from build123d import *

# Parameters (mm, degrees)
BOSS_EXTRUDE1_DEPTH               = 38.1
FILLET1_R                         = 5.08
SKETCH8_R                         = 1.7499965
SKETCH8_R_2                       = 1.75
CUT_EXTRUDE2_DEPTH                = 7.62
F_1_8_0_15_DOWEL_HOLE1_AT_2_COUNT = 2
F_1_8_0_15_DOWEL_HOLE1_AT_2_PITCH = 28.575
F_1_8_0_15_DOWEL_HOLE1_AT_3_COUNT = 2
F_1_8_0_15_DOWEL_HOLE1_AT_3_PITCH = 34.925
F_1_8_0_15_DOWEL_HOLE1_AT_4_COUNT = 2
F_1_8_0_15_DOWEL_HOLE1_AT_4_PITCH = 63.5
CUT_EXTRUDE3_DEPTH                = 4.7752
LPATTERN1_COUNT                   = 2
LPATTERN1_PITCH                   = 63.5
LPATTERN1_COUNT_DIR2              = 2
LPATTERN1_PITCH_DIR2              = 25.4
SKETCH16_W                        = 2.54
SKETCH16_H                        = 44.45
CUT_EXTRUDE4_DEPTH                = 7.62
SKETCH17_W                        = 76.2
SKETCH17_H                        = 19.05
CUT_EXTRUDE5_DEPTH                = 4.7752
SKETCH19_W                        = 12.6492
SKETCH19_H                        = 19.05
SKETCH19_W_2                      = 5.0292
BOSS_EXTRUDE6_DEPTH               = 4.7752
SKETCH22_R                        = 3.175
CGTEST1_DEPTH                     = 7.62


with BuildPart() as part:
    # Sketch1 → Boss-Extrude1 (new, symmetric)
    with BuildSketch(Plane.XY):
        Polygon((0, -24.348466848), (0, 114.923832009), (10.16, 114.923832009), (10.16, 122.543832009), (10.16, 142.863832009), (2.54, 142.863832009), (2.54, 122.543832009), (-7.62, 122.543832009), (-7.62, 114.923832009), (-7.62, -31.968466848), (2.54, -31.968466848), (2.54, -52.288466848), (10.16, -52.288466848), (10.16, -31.968466848), (10.16, -24.348466848), align=None)
    extrude(amount=BOSS_EXTRUDE1_DEPTH, both=True)

    # Fillet1
    fillet1_edges = [part.edges().sort_by_distance(p)[0] for p in [
        (0, -24.348466848, 0),
        (2.54, -31.968466848, 0),
        (0, 114.923832009, 0),
        (2.54, 122.543832009, 0),
        (-7.62, 122.543832009, 0),
        (-7.62, -31.968466848, 0),
    ]]
    fillet(fillet1_edges, radius=FILLET1_R - 0.0001)  # a hair under: the kernel refuses the full size

    # Sketch8 → Cut-Extrude2 (cut)
    with BuildSketch(Plane.ZY.offset(-2.54)):
        with Locations(Location((-31.75, 135.243832009, 0), (0, 0, 270))):
            Circle(SKETCH8_R)
        with Locations(Location((31.75, 135.243832009, 0), (0, 0, 270))):
            Circle(SKETCH8_R)
        with Locations(Location((-10.583333333, 135.243832009, 0), (0, 0, 270))):
            Circle(SKETCH8_R_2)
        with Locations(Location((10.583333333, 135.243832009, 0), (0, 0, 270))):
            Circle(SKETCH8_R_2)
    cut_extrude2 = extrude(amount=-CUT_EXTRUDE2_DEPTH, mode=Mode.SUBTRACT)

    # Mirror1: Cut-Extrude2 across plane
    add(cut_extrude2.mirror(Plane.ZX.offset(45.28768258)), mode=Mode.SUBTRACT)

    # Sketch11 → 1/8 (0.15) Dowel Hole1 (revolve, cut)
    with BuildSketch(Plane(origin=(-7.62, 27.82518258, 12.7), x_dir=(0, 0, 1), z_dir=(0, 1, 0))):
        Polygon((0, 0), (0, 8.764639479), (1.905, 7.62), (1.905, 0), align=None)
    f_1_8_0_15_dowel_hole1 = revolve(axis=Axis((-13.97, 27.82518258, 12.7), (1, 0, 0)), mode=Mode.SUBTRACT)

    # 1/8 (0.15) Dowel Hole1 at 2: 1/8 (0.15) Dowel Hole1 ×2
    with Locations(*[(0, -i * F_1_8_0_15_DOWEL_HOLE1_AT_2_PITCH, 0) for i in range(1, F_1_8_0_15_DOWEL_HOLE1_AT_2_COUNT)]):
        add(f_1_8_0_15_dowel_hole1, mode=Mode.SUBTRACT)

    # 1/8 (0.15) Dowel Hole1 at 3: 1/8 (0.15) Dowel Hole1 ×2
    with Locations(*[(0, i * F_1_8_0_15_DOWEL_HOLE1_AT_3_PITCH, 0) for i in range(1, F_1_8_0_15_DOWEL_HOLE1_AT_3_COUNT)]):
        add(f_1_8_0_15_dowel_hole1, mode=Mode.SUBTRACT)

    # 1/8 (0.15) Dowel Hole1 at 4: 1/8 (0.15) Dowel Hole1 ×2
    with Locations(*[(0, i * F_1_8_0_15_DOWEL_HOLE1_AT_4_PITCH, 0) for i in range(1, F_1_8_0_15_DOWEL_HOLE1_AT_4_COUNT)]):
        add(f_1_8_0_15_dowel_hole1, mode=Mode.SUBTRACT)

    # Sketch14 → Cut-Extrude3 (cut)
    with BuildSketch(Plane.ZY.offset(7.62)):
        Polygon((13.9954, 95.427086941), (11.4046, 95.427086941), (10.1092, 94.136177076), (10.1092, 59.947777076), (11.400109865, 58.652377076), (12.7, 58.652377076), (13.999890135, 58.652377076), (15.2908, 59.947777076), (15.2908, 94.136177076), align=None)
    cut_extrude3 = extrude(amount=-CUT_EXTRUDE3_DEPTH, mode=Mode.SUBTRACT)

    # LPattern1: Cut-Extrude3 2 × 2
    with Locations(*[(0, -i * LPATTERN1_PITCH, -j * LPATTERN1_PITCH_DIR2) for i in range(LPATTERN1_COUNT) for j in range(LPATTERN1_COUNT_DIR2) if (i, j) != (0, 0)]):
        add(cut_extrude3, mode=Mode.SUBTRACT)

    # Mirror2: 1/8 (0.15) Dowel Hole1 across plane
    add(f_1_8_0_15_dowel_hole1.mirror(Plane.XY), mode=Mode.SUBTRACT)

    # Mirror2 copy 1 sketch → Mirror2 copy 1 (revolve, cut)
    with BuildSketch(Plane(origin=(-7.62, -0.74981742, -12.7), x_dir=(0, 0, -1), z_dir=(0, 1, 0))):
        Polygon((0, 0), (0, -8.764639479), (1.905, -7.62), (1.905, 0), align=None)
    revolve(axis=Axis((-13.97, -0.74981742, -12.7), (-1, 0, 0)), mode=Mode.SUBTRACT)

    # Mirror2 copy 2 sketch → Mirror2 copy 2 (revolve, cut)
    with BuildSketch(Plane(origin=(-7.62, 62.75018258, -12.7), x_dir=(0, 0, -1), z_dir=(0, 1, 0))):
        Polygon((0, 0), (0, -8.764639479), (1.905, -7.62), (1.905, 0), align=None)
    revolve(axis=Axis((-13.97, 62.75018258, -12.7), (-1, 0, 0)), mode=Mode.SUBTRACT)

    # Mirror2 copy 3 sketch → Mirror2 copy 3 (revolve, cut)
    with BuildSketch(Plane(origin=(-7.62, 91.32518258, -12.7), x_dir=(0, 0, -1), z_dir=(0, 1, 0))):
        Polygon((0, 0), (0, -8.764639479), (1.905, -7.62), (1.905, 0), align=None)
    revolve(axis=Axis((-13.97, 91.32518258, -12.7), (-1, 0, 0)), mode=Mode.SUBTRACT)

    # Sketch16 → Cut-Extrude4 (cut)
    with BuildSketch(Plane.ZY.offset(7.62)):
        with Locations((3.81, 77.03768258)):
            Rectangle(SKETCH16_W, SKETCH16_H)
    cut_extrude4 = extrude(amount=-CUT_EXTRUDE4_DEPTH, mode=Mode.SUBTRACT)

    # Sketch17 → Cut-Extrude5 (cut)
    with BuildSketch(Plane.ZY.offset(7.62)):
        with Locations((0, 77.03768258)):
            Rectangle(SKETCH17_W, SKETCH17_H)
    cut_extrude5 = extrude(amount=-CUT_EXTRUDE5_DEPTH, mode=Mode.SUBTRACT)

    # Sketch19 → Boss-Extrude6 (add)
    with BuildSketch(Plane.ZY.offset(2.8448)):
        with Locations((-3.7846, 77.03768258)):
            Rectangle(SKETCH19_W, SKETCH19_H)
        with Locations((7.5946, 77.03768258)):
            Rectangle(SKETCH19_W_2, SKETCH19_H)
    boss_extrude6 = extrude(amount=BOSS_EXTRUDE6_DEPTH)

    # Mirror3: Cut-Extrude4, Cut-Extrude5, Boss-Extrude6 across plane
    add(cut_extrude4.mirror(Plane.ZX.offset(45.28768258)), mode=Mode.SUBTRACT)
    add(cut_extrude5.mirror(Plane.ZX.offset(45.28768258)), mode=Mode.SUBTRACT)
    add(boss_extrude6.mirror(Plane.ZX.offset(45.28768258)))

    # Sketch22 → CGTest1 (cut)
    with BuildSketch(Plane.ZY.offset(-2.54)):
        with Locations(Location((0, 135.243832009, 0), (0, 0, 270))):
            Circle(SKETCH22_R)
    extrude(amount=-CGTEST1_DEPTH, mode=Mode.SUBTRACT)


solid = part.part
Geometry: final body of the model. Coordinates: model frame, mm. A direction names the side the tool comes from. Round coordinates to 2 decimals unless told otherwise and drop trailing zeros. Loops run counter-clockwise (first coordinate to the right, second up) from the corner with the lowest first, then second, coordinate; pieces in that order, holes last. Notation, with made-up numbers: M 11.5,24 L 63.5,24 A30 cw 63.5,50 Z; hole C 79.25,6.25 d3. An arc over 180 degrees is marked long. Put each result on its own line as item: value. Start each with the question number.
(1) Section query C-C (y = 13). Return loops of the section in (x, z).
(2) Draft query along Z for faces 6 (the face through (-5, 86.563, 27)), 7 (the face through (-5, 14, -10.109)), 8 (the face through (-1, 47, 38.1)). Return one class per face: +Z half, -Z half, draft (parallel to the pull), parting line (faces both ways), or undercut.
(3) Section query B-B (z = -31.75). State how many separate pieces and enclosed holes the cut face has, then the cut area to 3 significant figures.
(4) Material intervals for line 1 along Z through (x, y) = (-5, 65); line 2 along Y through (x, z) = (6.75, -10.5); line 3 along Y through (x, z) = (5.75, 12), sorted ascending. Write a range as [from, to].
(5) Set-up query: faces 1 (the face through (-4, 77, 5.08)), 2 (the face through (-5, 4.013, 27)), 3 (the face through (1.45, 113.4, 0.53)), 4 (the face through (-5, 27, -15.291)), 5 (the face through (-5, 23.063, -27)). Return all of +Z, -Z, +X, -X, +Y, -Y with unobstructed straight access to the full face (end or side cutting, diameter ignored); none if empty.
(6) Contact query for flat-ended pins moving along their axis: pin 1 Ø3 at (x, z) = (-5, -13) entering from +Y; pin 2 Ø5 at (y, z) = (27.83, 12.7) entering from -X; pin 3 Ø8 at (y, z) = (17, -10) entering from +X. Output: stop coordinate, or through.
Findings below:
1. outline: M -7.62,-10.11 L -2.84,-10.11 L -2.84,-38.1 L 0,-38.1 L 0,2.54 L -7.62,2.54 Z; M -7.62,5.08 L 0,5.08 L 0,38.1 L -2.84,38.1 L -2.84,10.11 L -7.62,10.11 Z
2. face 6: draft
2. face 7: undercut
2. face 8: +Z half
3. separate pieces: 3
3. enclosed holes: 0
3. area: 1,420 mm2
4. line 1: z = [-38.1, -15.29], [-10.11, 2.54], [5.08, 10.11], [15.29, 38.1]
4. line 2: y = [-52.29, -46.42], [-42.92, -24.35], [114.92, 133.5], [136.99, 142.86]
4. line 3: y = [-52.29, -45.7], [-43.64, -24.35], [114.92, 134.22], [136.27, 142.86]
5. face 1: +X, -X
5. face 2: +Z, -X
5. face 3: +Z, -Z, +X
5. face 4: -X
5. face 5: -Z, -X
6. pin 1: stops at y = 122.45
6. pin 2: stops at x = -2.84
6. pin 3: stops at x = 0
